```python
from build123d import *

# Parameters (mm, degrees)
SKETCH1_R           = 7.5
BOSS_EXTRUDE1_DEPTH = 250
SKETCH2_R           = 5
CUT_EXTRUDE1_DEPTH  = 10
SKETCH3_R           = 9.435011435
SKETCH3_R_2         = 5
CUT_EXTRUDE2_DEPTH  = 19
SKETCH5_R           = 25.765699078
CUT_EXTRUDE3_DEPTH  = 221
SKETCH6_R           = 6.015267085
BOSS_EXTRUDE2_DEPTH = 10
SKETCH7_R           = 2.5
CUT_EXTRUDE4_DEPTH  = 10


with BuildPart() as part:
    # Sketch1 → Boss-Extrude1 (new body)
    with BuildSketch(Plane.XY):
        Circle(SKETCH1_R)
    extrude(amount=BOSS_EXTRUDE1_DEPTH)

    # Sketch2 → Cut-Extrude1 (cut)
    with BuildSketch(Plane.XY):
        Circle(SKETCH2_R)
    extrude(amount=CUT_EXTRUDE1_DEPTH, mode=Mode.SUBTRACT)

    # Sketch3 → Cut-Extrude2 (cut)
    with BuildSketch(Plane(origin=(0, 0, 10), x_dir=(-1, 0, 0), z_dir=(0, 0, -1))):
        Circle(SKETCH3_R)
        Circle(SKETCH3_R_2, mode=Mode.SUBTRACT)
    extrude(amount=-CUT_EXTRUDE2_DEPTH, mode=Mode.SUBTRACT)


with BuildPart() as cut_extrude2_piece_1:
    # of the separate pieces the step leaves, piece 1, a body of its own (cut_extrude2_pieces)
    add(part.part.solids().sort_by_distance((7.5, 0, 29))[0])

    # Sketch5 → Cut-Extrude3 (cut)
    with BuildSketch(Plane(origin=(0, 0, 29), x_dir=(-1, 0, 0), z_dir=(0, 0, -1))):
        Circle(SKETCH5_R)
    extrude(amount=-CUT_EXTRUDE3_DEPTH, mode=Mode.SUBTRACT)



with BuildPart() as cut_extrude2_piece_2:
    # of the separate pieces the step leaves, piece 2, a body of its own (cut_extrude2_pieces)
    add(part.part.solids().sort_by_distance((7.5, 0, 0))[0])


with BuildPart() as cut_extrude2_piece_1_1:
    add(cut_extrude2_piece_1.part)

    add(cut_extrude2_piece_2.part)  # Boss-Extrude2 merges Cut-Extrude2 piece 2
    # Sketch6 → Boss-Extrude2 (add)
    with BuildSketch(Plane(origin=(0, 0, 10), x_dir=(-1, 0, 0), z_dir=(0, 0, -1))):
        Circle(SKETCH6_R)
    extrude(amount=BOSS_EXTRUDE2_DEPTH)

    # Sketch7 → Cut-Extrude4 (cut)
    with BuildSketch(Plane.XY.offset(29)):
        Circle(SKETCH7_R)
    extrude(amount=-CUT_EXTRUDE4_DEPTH, mode=Mode.SUBTRACT)


solid = cut_extrude2_piece_1_1.part
```
Model file for the job. Use its own axes, mm. A direction names the side the tool comes from. Coordinates: 2 decimals unless noted, no trailing zeros. Loops run counter-clockwise (first coordinate to the right, second up) from the corner with the lowest first, then second, coordinate; pieces in that order, holes last. Notation, with made-up numbers: (-17.5, 49) - (37.5, 49) arc R21 ccw to (37.5, 79) - close; hole circle Ø10 at (-31.5, 78.25). An arc over 180 degrees is marked (long way). Answer as a JSON object with one key per item and string values. Group by question number.
(1) Probe line 1 along Y through (x, z) = (0, 24); line 2 along Z through (x, y) = (0, 0.75); line 3 along Z through (x, y) = (-4, -5.75). List the from-to ranges inside material, lowest first.
(2) Cut at D-D (z = 6.25). Give the cut face in (x, y), then the cut area to 3 significant figures.
(3) Cut at B-B (x = 0). Give the cut face in (y, z).
(4) Two-plate mould, pull along Y, no slides. Class faces 3 (the face through (-7.493, 0.33, 4.93)), 4 (the face through (-2, -2, 29)), 5 (the face through (-0.54, -2.44, 24.07)): released by +Y, released by -Y, zero draft, split by the parting line, or undercut.
(5) Tool access for faces 1 (the face through (-2, -5, 10)), 2 (the face through (0, 0, 0)): list every direction of +Z, -Z, +X, -X, +Y, -Y with a clear straight run to the whole face (end or side of a thin tool).
(6) Flat gauge pins, fed straight in: pin 1 (2 mm diameter, centred on y = -0.5, z = 15, fed in from +X); pin 2 (2 mm diameter, centred on y = 1.5, z = 19, fed in from -X); pin 3 (6 mm diameter, centred on y = 4, z = 20, fed in from +X). Where does each tip first touch, or does it go through?
(7) Cut at A-A (z = 22.75). Give the cut face in (x, y), then the cut area to 3 significant figures.
Geometry says:
{
 "1": {"line 1": "y = -5 to -2.5, 2.5 to 5", "line 2": "z = 0 to 19", "line 3": "z = 0 to 10"},
 "2": {"outline": "circle Ø15 at (0, 0)", "area": "177 mm^2"},
 "3": {"outline": "(-7.5, 0) - (7.5, 0) - (7.5, 10) - (5, 10) - (5, 29) - (2.5, 29) - (2.5, 19) - (-2.5, 19) - (-2.5, 29) - (-5, 29) - (-5, 10) - (-7.5, 10) - close"},
 "4": {"face 3": "split by the parting line", "face 4": "zero draft", "face 5": "undercut"},
 "5": {"face 1": "+Z", "face 2": "-Z, +X, -X, +Y, -Y"},
 "6": {"pin 1": "stops at x = 5", "pin 2": "stops at x = -4.97", "pin 3": "stops at x = 4.9"},
 "7": {"outline": "circle Ø10 at (0, 0); hole circle Ø5 at (0, 0)", "area": "58.9 mm^2"}
}
